Part model, mm, in its own coordinate system. Face numbers are marked on the shaded views. Coordinates: 2 decimals unless noted, no trailing zeros. Loops run counter-clockwise (first coordinate to the right, second up) from the corner with the lowest first, then second, coordinate; pieces in that order, holes last. Notation, with made-up numbers: (60.5, 4.25) - (113.5, 4.25) arc R13 ccw to (113.5, 29.25) - close; hole circle Ø6 at (26.25, 34.25). An arc over 180 degrees is marked (long way). Use a Markdown table: item, result. Add a question column.
1) Drop flat-ended pins along their axis: P1, Ø1, axis at y = -3, z = 1.5, coming from the +X side; P2, Ø0.6, axis at x = 12.5, z = 1.5, coming from the -Y side. Give the stop position or say it passes through.
2) Probe probe 1 along X at (y, z) = (-1.5, 0.7); probe 2 along Y at (x, z) = (-5.5, 0.6); probe 3 along Y at (x, z) = (-0.5, 0.5). List the from-to ranges inside material, lowest first. Write a range as [from, to].
3) Band-saw the part on A-A (y = 8). Give the cut face in (x, z), plus the area to 3 significant figures.
4) Pull direction Y, two halves, no side cores. Call the marked faces 1 and 2: +Y half, -Y half, draft (parallel to the pull), parting line (faces both ways), or undercut.
5) Band-saw the part on C-C (x = -6). Give the cut face in (y, z), plus the area to 3 significant figures.
6) Band-saw the part on D-D (x = 0.5). Give the cut face in (y, z), plus the area to 3 significant figures.
7) Band-saw the part on B-B (z = 0.85). Give the cut face in (x, y).
from build123d import *

# Parameters (mm, degrees)
SKETCH1_R           = 1
BOSS_EXTRUDE1_DEPTH = 2


with BuildPart() as part:
    # Sketch1 → Boss-Extrude1 (new body)
    with BuildSketch(Plane.XY):
        with BuildLine():
            Line((9.9326669, -1), (14.865841105, -1))
            Line((14.865841105, -1), (14.865841105, 10))
            ThreePointArc((14.865841105, 10), (13.401375011, 13.535533906), (9.865841105, 15))
            Line((9.865841105, 15), (-9.865841105, 15))
            ThreePointArc((-9.865841105, 15), (-13.401375011, 13.535533906), (-14.865841105, 10))
            Line((-14.865841105, 10), (-14.865841105, -1))
            Line((-14.865841105, -1), (-7.151873985, -1))
            Line((-7.151873985, -1), (-7.151873985, -5))
            Line((-7.151873985, -5), (-2.151873985, -5))
            Line((-2.151873985, -5), (-2.151873985, -1))
            Line((-2.151873985, -1), (1.9326669, -1))
            Line((1.9326669, -1), (1.9326669, -5))
            Line((1.9326669, -5), (9.9326669, -5))
            Line((9.9326669, -5), (9.9326669, -1))
        make_face()
        with Locations((-5.434158895, 8)):
            Circle(SKETCH1_R, mode=Mode.SUBTRACT)
    extrude(amount=BOSS_EXTRUDE1_DEPTH)


solid = part.part
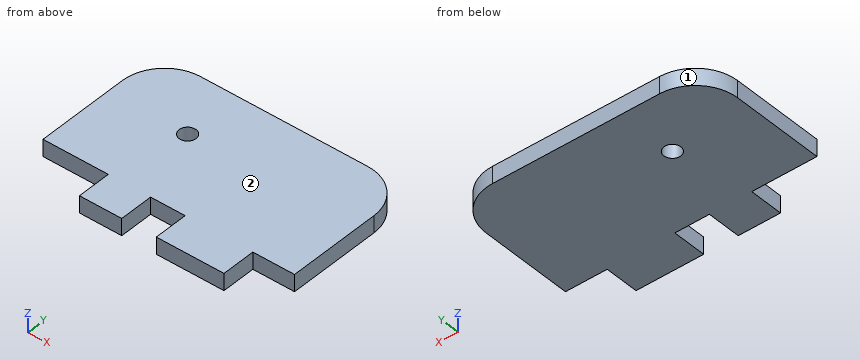
Answer block:
| question | item | result |
|---|---|---|
| 1 | P1 | x = 9.93 |
| 1 | P2 | y = -1 |
| 2 | probe 1 | [-7.15, -2.15], [1.93, 9.93] |
| 2 | probe 2 | [-5, 7], [9, 15] |
| 2 | probe 3 | [-1, 15] |
| 3 | outline | (-14.87, 0) - (-6.43, 0) - (-6.43, 2) - (-14.87, 2) - close; (-4.43, 0) - (14.87, 0) - (14.87, 2) - (-4.43, 2) - close |
| 3 | area | 55.5 mm2 |
| 4 | face 1 | +Y half |
| 4 | face 2 | draft |
| 5 | outline | (-5, 0) - (7.18, 0) - (7.18, 2) - (-5, 2) - close; (8.82, 0) - (15, 0) - (15, 2) - (8.82, 2) - close |
| 5 | area | 36.7 mm2 |
| 6 | outline | (-1, 0) - (15, 0) - (15, 2) - (-1, 2) - close |
| 6 | area | 32.0 mm2 |
| 7 | outline | (-14.87, -1) - (-7.15, -1) - (-7.15, -5) - (-2.15, -5) - (-2.15, -1) - (1.93, -1) - (1.93, -5) - (9.93, -5) - (9.93, -1) - (14.87, -1) - (14.87, 10) arc R5 ccw to (9.87, 15) - (-9.87, 15) arc R5 ccw to (-14.87, 10) - close; hole circle Ø2 at (-5.43, 8) |
